Build history of the part. All positions in model axes, mm. A direction names the side the tool comes from. Give positions to 0.01 mm unless a question says otherwise; leave off trailing zeros. Order: outer loops, then holes, each group sorted by start corner. A loop starts at its lowest first (then second) coordinate and runs counter-clockwise, first axis right, second up. Notation, with made-up numbers: (69.5, 74) - (127.5, 74) arc R6 ccw to (127.5, 79) - close; hole circle Ø11 at (23.5, 13). An arc over 180 degrees is marked (long way). One line per item, written item: value.
```python
from build123d import *
from build123d.topology import SkipClean

# Parameters (mm, degrees)
SKETCH2_W           = 44
SKETCH2_H           = 31
SKETCH2_H_2         = 32
SKETCH2_W_2         = 60
SKETCH2_H_3         = 73
BOSS_EXTRUDE1_DEPTH = 30
SKETCH3_R           = 45
SKETCH3_R_2         = 35
BOSS_EXTRUDE2_DEPTH = 120
FILLET1_R           = 5
SKETCH6_R           = 35
CUT_EXTRUDE1_DEPTH  = 120
FILLET2_R           = 5


with BuildPart() as part:
    # Sketch2 → Boss-Extrude1 (new body)
    with BuildSketch(Plane.XY):
        Polygon((22.104569931, 160.536781585), (102.104569931, 160.536781585), (102.104569931, -130.963218415), (-91.895430069, -130.963218415), (-91.895430069, -57.963218415), align=None)
        with Locations((70.104569931, 135.036781585)):
            Rectangle(SKETCH2_W, SKETCH2_H, mode=Mode.SUBTRACT)
        with Locations((70.104569931, -104.963218415)):
            Rectangle(SKETCH2_W, SKETCH2_H_2, mode=Mode.SUBTRACT)
        with Locations((-59.895430069, -104.963218415)):
            Rectangle(SKETCH2_W, SKETCH2_H_2, mode=Mode.SUBTRACT)
        with Locations((5.104569931, -83.895986651)):
            Rectangle(SKETCH2_W_2, SKETCH2_H_3, mode=Mode.SUBTRACT)
    extrude(amount=BOSS_EXTRUDE1_DEPTH)

    # Sketch3 → Boss-Extrude2 (add)
    with BuildSketch(Plane(origin=(0, 0, 0), x_dir=(-1, 0, 0), z_dir=(0, 0, -1))):
        with Locations((-5.104569931, 22.786781585)):
            Circle(SKETCH3_R)
        with Locations((-5.104569931, 22.786781585)):
            Circle(SKETCH3_R_2, mode=Mode.SUBTRACT)
    extrude(amount=BOSS_EXTRUDE2_DEPTH)

    # Fillet1
    fillet1_edges = [part.edges().sort_by_distance(p)[0] for p in [
        (92.104569931, 119.536781585, 15),
        (92.104569931, 150.536781585, 15),
        (48.104569931, 150.536781585, 15),
        (48.104569931, 119.536781585, 15),
    ]]
    fillet(fillet1_edges, radius=FILLET1_R)

    # Sketch6 → Cut-Extrude1 (cut)
    with SkipClean():  # the faces are left unmerged after this step: merging them gives an invalid solid
        with BuildSketch(Plane.XY.offset(30)):
            with Locations((5.104569931, 22.786781585)):
                Circle(SKETCH6_R)
        extrude(amount=-CUT_EXTRUDE1_DEPTH, mode=Mode.SUBTRACT)
    add(part.part.scale(1), mode=Mode.REPLACE)  # the faces are merged on a copy

    # Fillet2
    fillet2_edges = [part.edges().sort_by_distance(p)[0] for p in [
        (50.104569931, 22.786781585, 0),
    ]]
    fillet(fillet2_edges, radius=FILLET2_R)


solid = part.part
```
(1) Drill centre lines: line 1 (Z direction, x = -23, y = -25); line 2 (X direction, y = 34, z = -68.5); line 3 (X direction, y = 38.5, z = -33). Where is each one in solid material? Low to high.
Completed:
line 1: 0 to 30
line 2: -38.48 to -28.05, 38.26 to 48.69
line 3: -37.06 to -26.17, 36.38 to 47.27
(2) Pull direction Y, two halves, no side cores. Call faces 4 (the face through (6, -130.963, 15)), 5 (the face through (102.105, 17, 15)), 6 (the face through (70, 119.537, 15)): +Y half, -Y half, draft (parallel to the pull), parting line (faces both ways), or undercut.
Completed:
face 4: -Y half
face 5: draft
face 6: undercut
(3) Slice it at D-D, the plane z = -34.5. Give the cut face in (x, y).
Completed:
outline: circle Ø90 at (5.1, 22.79); hole circle Ø70 at (5.1, 22.79)
(4) Slice it at A-A, the plane y = -103.5. Give the cut face in (x, z), and give its area (3 significant figures).
Completed:
outline: (-91.9, 0) - (-81.9, 0) - (-81.9, 30) - (-91.9, 30) - close; (-37.9, 0) - (-24.9, 0) - (-24.9, 30) - (-37.9, 30) - close; (35.1, 0) - (48.1, 0) - (48.1, 30) - (35.1, 30) - close; (92.1, 0) - (102.1, 0) - (102.1, 30) - (92.1, 30) - close
area: 1,380 mm²
(5) Pin check, flat tips, straight feed: P1, Ø2, axis at x = 47, y = 73, coming from the -Z side; P2, Ø6, axis at y = -8.5, z = -24.5, coming from the -X side; P3, Ø17, axis at y = 130.5, z = 8.5, coming from the -X side. Stop position of each tip, or through.
Completed:
P1: z = 0
P2: x = -29.89
P3: x = 2
(6) 3-axis set-ups, long thin cutter, end or side, ignore diameter. For faces 1 (the face through (-35.69, 49.76, 14.79)), 2 (the face through (70, -120.963, 15)), 3 (the face through (14.86, -21.143, -61.563)): which of +Z, -Z, +X, -X, +Y, -Y reach the whole face in a straight line?
Completed:
face 1: +Z, -Z, -X, +Y
face 2: +Z, -Z
face 3: -Z
(7) Slice it at C-C, the plane z = 16. Give the cut face in (x, y).
Completed:
outline: (-91.9, -130.96) - (102.1, -130.96) - (102.1, 160.54) - (22.1, 160.54) - (-91.9, -57.96) - close; hole (-81.9, -120.96) - (-37.9, -120.96) - (-37.9, -88.96) - (-81.9, -88.96) - close; hole circle Ø70 at (5.1, 22.79); hole (-24.9, -120.4) - (35.1, -120.4) - (35.1, -47.4) - (-24.9, -47.4) - close; hole (48.1, -120.96) - (92.1, -120.96) - (92.1, -88.96) - (48.1, -88.96) - close; hole (48.1, 124.54) arc R5 ccw to (53.1, 119.54) - (87.1, 119.54) arc R5 ccw to (92.1, 124.54) - (92.1, 145.54) arc R5 ccw to (87.1, 150.54) - (53.1, 150.54) arc R5 ccw to (48.1, 145.54) - close
(8) Slice it at B-B, the plane x = -61. Give the cut face in (y, z), and give its area (3 significant figures).
Completed:
outline: (-130.96, 0) - (-120.96, 0) - (-120.96, 30) - (-130.96, 30) - close; (-88.96, 0) - (1.25, 0) - (1.25, 30) - (-88.96, 30) - close
area: 3,010 mm²
